from build123d import *

# Parameters (mm, degrees)
SKETCH1_R             = 3.424139869
BOSS_EXTRUDE1_DEPTH   = 10
BOSS_EXTRUDE1_2_DEPTH = 10
SKETCH2_W             = 106.866754861
SKETCH2_H             = 90
BOSS_EXTRUDE2_DEPTH   = 5
SKETCH3_W             = 107
SKETCH3_H             = 5
BOSS_EXTRUDE3_DEPTH   = 10
SKETCH4_W             = 107
SKETCH4_H             = 8
BOSS_EXTRUDE4_DEPTH   = 10


with BuildPart() as part:
    # Sketch1 → Boss-Extrude1 (new body)
    with BuildSketch(Plane.XY):
        with Locations((-27.5, 9)):
            Circle(SKETCH1_R)
    extrude(amount=BOSS_EXTRUDE1_DEPTH)



with BuildPart() as body_2:
    # Sketch1 → Boss-Extrude1 2 (new body)
    with BuildSketch(Plane.XY):
        with Locations((23.5, -7)):
            Circle(SKETCH1_R)
    extrude(amount=BOSS_EXTRUDE1_2_DEPTH)


with BuildPart() as part_1:
    add(part.part)

    add(body_2.part)  # Boss-Extrude2 merges body 2
    # Sketch2 → Boss-Extrude2 (add)
    with BuildSketch(Plane(origin=(0, 0, 0), x_dir=(-1, 0, 0), z_dir=(0, 0, -1))):
        with Locations((0.066622569, -8)):
            Rectangle(SKETCH2_W, SKETCH2_H)
    extrude(amount=BOSS_EXTRUDE2_DEPTH)

    # Sketch3 → Boss-Extrude3 (add)
    with BuildSketch(Plane.XY):
        with Locations((0, -50.5)):
            Rectangle(SKETCH3_W, SKETCH3_H)
    extrude(amount=BOSS_EXTRUDE3_DEPTH)

    # Sketch4 → Boss-Extrude4 (add)
    with BuildSketch(Plane.XY):
        with Locations((0, -34)):
            Rectangle(SKETCH4_W, SKETCH4_H)
    extrude(amount=BOSS_EXTRUDE4_DEPTH)


solid = part_1.part
Input: part model. Units: mm. Frame: model coordinates. A direction names the side the tool comes from. Give positions to 0.01 mm unless a question says otherwise; leave off trailing zeros. Write each loop counter-clockwise with the first axis right and the second up, starting at its lowest first coordinate (ties: lowest second). Pieces come first, ordered by that corner, then holes. Notation, with made-up numbers: (16.25, 9) -> (27.25, 9) arc R19 cw to (27.25, 40) -> close; hole circle Ø6 at (81, 33). An arc over 180 degrees is marked (long way). Use one line per item in the form item = value. Start each with the question number.
1) Pin query (flat end, axial travel): pin 1 (5 mm diameter, centred on x = -25.5, z = 4.5, fed in from +Y); pin 2 (5 mm diameter, centred on x = 20, y = -41.5, fed in from +Z); pin 3 (2.5 mm diameter, centred on y = -24.5, z = -3, fed in from +X). Return the tip coordinate at first contact, or that it passes through.
2) Ray query, probe 1 along Y at (x, z) = (32, 2.75); probe 2 along Y at (x, z) = (24, 2.5); probe 3 along Y at (x, z) = (21, 5). Return the intervals inside material, ascending. Write a range as from..to.
3) Section query D-D on x = 23.5. Return the cut outline in (y, z).
4) Draft query along Y for faces 1 (the cylindrical face through (20.08, -6.85, 4.93)), 2 (the flat face through (-1, -38, 5)), 3 (the flat face through (-1, -53, 2)), 4 (the flat face through (53.367, -9, -2)). Return one class per face: pulls with the +Y half, pulls with the -Y half, needs draft (parallel to the pull), parting line crosses it, or undercut.
5) Set-up query: faces 5 (the flat face through (1, -7, -5)), 6 (the flat face through (-1, -48, 5)), 7 (the cylindrical face through (-28.242, 5.657, 4.93)). Return all of +Z, -Z, +X, -X, +Y, -Y with unobstructed straight access to the full face (end or side cutting, diameter ignored); none if empty.
6) Section query A-A on z = 6.25. Return the cut outline in (x, y), then the cut area to 3 significant figures.
7) Section query C-C on y = 9. Return the cut outline in (x, z).
8) Section query B-B on x = -15. Return the cut outline in (y, z).
Outcome:
q1.pin_1 = 12.42
q1.pin_2 = 0
q1.pin_3 = 53.37
q2.probe_1 = -53..-48, -38..-30
q2.probe_2 = -53..-48, -38..-30, -10.39..-3.61
q2.probe_3 = -53..-48, -38..-30, -9.34..-4.66
q3.outline = (-53, -5) -> (37, -5) -> (37, 0) -> (-3.58, 0) -> (-3.58, 10) -> (-10.42, 10) -> (-10.42, 0) -> (-30, 0) -> (-30, 10) -> (-38, 10) -> (-38, 0) -> (-48, 0) -> (-48, 10) -> (-53, 10) -> close
q4.face_1 = undercut
q4.face_2 = undercut
q4.face_3 = pulls with the -Y half
q4.face_4 = needs draft
q5.face_5 = -Z, +X, -X, +Y, -Y
q5.face_6 = +Z, +X, -X
q5.face_7 = +Z
q6.outline = (-53.5, -53) -> (53.5, -53) -> (53.5, -48) -> (-53.5, -48) -> close; (-53.5, -38) -> (53.5, -38) -> (53.5, -30) -> (-53.5, -30) -> close; circle Ø6.85 at (-27.5, 9); circle Ø6.85 at (23.5, -7)
q6.area = 1,460 mm^2
q7.outline = (-53.5, -5) -> (53.37, -5) -> (53.37, 0) -> (-24.08, 0) -> (-24.08, 10) -> (-30.92, 10) -> (-30.92, 0) -> (-53.5, 0) -> close
q8.outline = (-53, -5) -> (37, -5) -> (37, 0) -> (-30, 0) -> (-30, 10) -> (-38, 10) -> (-38, 0) -> (-48, 0) -> (-48, 10) -> (-53, 10) -> close
